from build123d import *

# Parameters (mm, degrees)
F2_R     = 16.51
F2_R_2   = 12.7
F4_R     = 19.05
F4_R_2   = 12.7
F5_DEPTH = 2.54
F6_R     = 19.05
F6_R_2   = 12.7
F7_DEPTH = 2.54


with BuildPart() as f3:
    # F3: sweep along a path in F0
    with BuildLine(Plane.XZ) as f3_path:
        Line((12.7, 0), (0, 0))
        ThreePointArc((0, 0), (-35.921024, 14.878976), (-50.8, 50.8))
        Line((-50.8, 50.8), (-50.8, 63.5))
    # F2 (on offset) → F3 (sweep)
    with BuildSketch(Plane.YZ.offset(12.7)):
        Circle(F2_R)
        Circle(F2_R_2, mode=Mode.SUBTRACT)
    sweep(path=f3_path.line)

    # F4 (on face) → F5 (join)
    with BuildSketch(Plane.YZ.offset(12.7)):
        Circle(F4_R)
        Circle(F4_R_2, mode=Mode.SUBTRACT)
    extrude(amount=-F5_DEPTH)

    # F6 (on face) → F7 (join)
    with BuildSketch(Plane.XY.offset(63.5)):
        with Locations((-50.8, 0)):
            Circle(F6_R)
        with Locations((-50.8, 0)):
            Circle(F6_R_2, mode=Mode.SUBTRACT)
    extrude(amount=-F7_DEPTH)


solid = f3.part
The listing builds one solid part. Answer for the finished solid, in the listing's coordinates (mm). A direction names the side the tool comes from. Give positions to 0.01 mm unless a question says otherwise; leave off trailing zeros. Order: outer loops, then holes, each group sorted by start corner. A loop starts at its lowest first (then second) coordinate and runs counter-clockwise, first axis right, second up. Notation, with made-up numbers: (24.25, -26) - (75.25, -26) arc R26 cw to (75.25, 8) - close; hole circle Ø10 at (22.5, 86). An arc over 180 degrees is marked (long way). Answer as CSV lines item,"result".
Q1. A cutting plane is placed at B-B, the plane z = 18. Count the separate pieces of the cut face and the enclosed holes in it, and give its area (3 significant figures).
Answer key:
separate pieces,"2"
enclosed holes,"1"
area,"558 mm^2"
Q2. Each of these flat-tipped pins is pushed along its axis until it touches: pin 1 Ø5 at (x, y) = (-19.5, 5.5) entering from -Z; pin 2 Ø1.5 at (y, z) = (10.5, 20) entering from -X; pin 3 Ø4 at (y, z) = (3, 35) entering from -X. Where does it stop, or does it pass through?
Answer key:
pin 1,"stops at z = -13.69"
pin 2,"stops at x = -56.36"
pin 3,"stops at x = -65.7"
Q3. Determine the mould class of faces 1 (the face through (11.45, -15.12, -11.59)), 2 (the face through (-33.203, -7.296, 62.248)), 3 (the face through (10.16, -6, 16)) for opening direction X: pulls with the +X half, pulls with the -X half, needs draft (parallel to the pull), parting line crosses it, or undercut.
Answer key:
face 1,"needs draft"
face 2,"parting line crosses it"
face 3,"undercut"
Q4. A cutting plane is placed at A-A, the plane x = 1. Determine the outline of the cut face in (y, z).
Answer key:
outline,"circle Ø33.02 at (0, 0); hole circle Ø25.4 at (0, 0)"
Q5. Straight lines are drawn through the part: L1, parallel to Y at x = 8.5, z = 0; L2, parallel to Z at x = -30.5, y = 8.5. For each, find the intervals that lie inside material, in ascending order.
Answer key:
L1,"y = -16.51 to -12.7, 12.7 to 16.51"
L2,"z = -6.55 to -1.14, 22.86 to 30.49"
Q6. Which of the six approach directions +Z, -Z, +X, -X, +Y, -Y give full straight-line access (tool end or side, diameter ignored) to faces 4 (the face through (6.26, -2.75, 12.4)), 5 (the face through (-57, 16, 60.96)), 6 (the face through (12.7, 4, -12.4))?
Answer key:
face 4,"+X"
face 5,"none"
face 6,"+Z, -Z, +X, +Y, -Y"
